from build123d import *

# Parameters (mm, degrees)
SKETCH1_W           = 12
SKETCH1_H           = 10
BOSS_EXTRUDE1_DEPTH = 7
SKETCH2_R           = 1.6
CUT_EXTRUDE1_DEPTH  = 4
SKETCH3_W           = 5.6
SKETCH3_H           = 2.6
CUT_EXTRUDE2_DEPTH  = 7
FILLET1_R           = 6
FILLET2_R           = 1
FILLET3_R           = 1
FILLET4_R           = 0.5


with BuildPart() as part:
    # Sketch1 → Boss-Extrude1 (new body)
    with BuildSketch(Plane(origin=(0, 0, 0), x_dir=(1, 0, 0), z_dir=(0, 1, 0))):
        with Locations((6, 5)):
            Rectangle(SKETCH1_W, SKETCH1_H)
    extrude(amount=BOSS_EXTRUDE1_DEPTH)

    # Sketch2 → Cut-Extrude1 (cut)
    with BuildSketch(Plane(origin=(0, 7, 0), x_dir=(1, 0, 0), z_dir=(0, 1, 0))):
        with Locations(Location((6, 4, 0), (0, 0, 270))):
            Circle(SKETCH2_R)
    extrude(amount=-CUT_EXTRUDE1_DEPTH, mode=Mode.SUBTRACT)

    # Sketch3 → Cut-Extrude2 (cut)
    with BuildSketch(Plane.XY):
        with Locations((6, 4.5)):
            Rectangle(SKETCH3_W, SKETCH3_H)
    extrude(amount=-CUT_EXTRUDE2_DEPTH, mode=Mode.SUBTRACT)

    # Fillet1
    fillet1_edges = [part.edges().sort_by_distance(p)[0] for p in [
        (0, 3.5, -10),
        (12, 3.5, -10),
    ]]
    fillet(fillet1_edges, radius=FILLET1_R - 0.0001)  # a hair under: the kernel refuses the full size

    # Fillet2
    fillet2_edges = [part.edges().sort_by_distance(p)[0] for p in [
        (0, 0, -2.00005),
        (10.242669976, 0, -8.242669976),
        (1.757330024, 0, -8.242669976),
        (12, 0, -2.00005),
    ]]
    fillet(fillet2_edges, radius=FILLET2_R)

    # Fillet3
    fillet3_edges = [part.edges().sort_by_distance(p)[0] for p in [
        (6, 0, 0),
        (11.707106781, 0.292893219, 0),
        (0.292893219, 0.292893219, 0),
        (12, 4, 0),
        (0, 4, 0),
    ]]
    fillet(fillet3_edges, radius=FILLET3_R)

    # Fillet4
    fillet4_edges = [part.edges().sort_by_distance(p)[0] for p in [
        (0, 7, -2.50005),
        (10.242669976, 7, -8.242669976),
        (1.757330024, 7, -8.242669976),
        (6, 7, 0),
        (12, 7, -2.50005),
        (11.707106781, 7, -0.292893219),
        (0.292893219, 7, -0.292893219),
    ]]
    fillet(fillet4_edges, radius=FILLET4_R)


solid = part.part
Geometry: final body of the model. Coordinates: model frame, mm. A direction names the side the tool comes from. Coordinates: 2 decimals unless noted, no trailing zeros. Write each loop counter-clockwise with the first axis right and the second up, starting at its lowest first coordinate (ties: lowest second). Pieces come first, ordered by that corner, then holes. Notation, with made-up numbers: (-28.5, -10.5) - (7.5, -10.5) arc R20 ccw to (7.5, 2.5) - close; hole circle Ø11 at (23, 42). An arc over 180 degrees is marked (long way). Return JSON: item names as keys, results as strings.
Item 1: Pin query (flat end, axial travel): pin 1 Ø1.5 at (y, z) = (3.5, -6) entering from -X; pin 2 Ø0.8 at (x, y) = (6.5, 4) entering from +Z. Return the tip coordinate at first contact, or that it passes through.
Completed:
{"pin 1": "stops at x = 0.13", "pin 2": "stops at z = -7"}
Item 2: Pull-direction query (X, two-part tool) for faces 1 (the face through (6, 3, 0)), 2 (the face through (0.285, 0.301, -2.521)), 3 (the face through (3.2, 4, -3)); classes: +X half, -X half, draft (parallel to the pull), parting line (faces both ways), or undercut.
Completed:
{"face 1": "draft", "face 2": "-X half", "face 3": "undercut"}
Item 3: Reachability of faces 4 (the face through (4.44, 6.41, -4.35)), 5 (the face through (4.7, 3.2, -2.7)), 6 (the face through (0, 4, -2)) from +Z, -Z, +X, -X, +Y, -Y: full face, straight path, thin tool, end or side. Return the list, or none.
Completed:
{"face 4": "+Y", "face 5": "+Z", "face 6": "+Z, -Z, -X, +Y, -Y"}
Item 4: Section query D-D (z = -3). Output: boundary loops of the cut face in (x, y), and give its area (3 significant figures).
Completed:
{"outline": "(0, 1) arc R1 ccw to (1, 0) - (11, 0) arc R1 ccw to (12, 1) - (12, 6.5) arc R0.5 ccw to (11.5, 7) - (7.25, 7) - (7.25, 5.8) - (8.8, 5.8) - (8.8, 3.2) - (7.25, 3.2) - (7.25, 3) - (4.75, 3) - (4.75, 3.2) - (3.2, 3.2) - (3.2, 5.8) - (4.75, 5.8) - (4.75, 7) - (0.5, 7) arc R0.5 ccw to (0, 6.5) - close", "area": "65.4 mm2"}
Item 5: Line query: L1, parallel to Y at x = 5.25, z = -6.75; L2, parallel to X at y = 4.5, z = -1.5; L3, parallel to X at y = 3.15, z = -4. Output: solid intervals per line, ascending.
Completed:
{"L1": "y = 0 to 3.2, 5.8 to 7", "L2": "x = 0 to 3.2, 8.8 to 12", "L3": "x = 0 to 4.4, 7.6 to 12"}
Item 6: Section query A-A (z = -1.5). Output: boundary loops of the cut face in (x, y), and give its area (3 significant figures).
Completed:
{"outline": "(0, 1) arc R1 ccw to (1, 0) - (11, 0) arc R1 ccw to (12, 1) - (12, 6.5) arc R0.5 ccw to (11.5, 7) - (0.5, 7) arc R0.5 ccw to (0, 6.5) - close; hole (3.2, 3.2) - (8.8, 3.2) - (8.8, 5.8) - (3.2, 5.8) - close", "area": "68.9 mm2"}
